Build history of the part. All positions in model axes, mm. A direction names the side the tool comes from. Round coordinates to 2 decimals unless told otherwise and drop trailing zeros. Write each loop counter-clockwise with the first axis right and the second up, starting at its lowest first coordinate (ties: lowest second). Pieces come first, ordered by that corner, then holes. Notation, with made-up numbers: (84.25, 46) -> (107.25, 46) arc R16 cw to (107.25, 70) -> close; hole circle Ø1 at (-34.75, 32). An arc over 180 degrees is marked (long way). One line per question, with ' | ' between items.
from build123d import *

# Parameters (mm, degrees)
SKETCH1_W                    = 275
SKETCH1_H                    = 33
BOSS_EXTRUDE1_DEPTH          = 12
CUT_EXTRUDE1_REACH           = 141.005
SKETCH2_R                    = 7
BOSS_EXTRUDE2_DEPTH          = 12
CUT_EXTRUDE3_REACH           = 264.774
SKETCH5_W                    = 14
SKETCH5_H                    = 6
FILLET1_R                    = 2
SKETCH17_W                   = 5
SKETCH17_H                   = 24
CUT_EXTRUDE9_DEPTH           = 6.5
CUT_EXTRUDE4_REACH           = 264.774
SKETCH6_W                    = 12
SKETCH6_H                    = 30
F_5_0_5_DIAMETER_HOLE2_D     = 5
F_5_0_5_DIAMETER_HOLE1_D     = 5
F_5_0_5_DIAMETER_HOLE1_DEPTH = 12
F_5_0_5_DIAMETER_HOLE1_TIP   = 1.502151548
FILLET2_R                    = 10
CUT_EXTRUDE5_REACH           = 264.774
CUT_EXTRUDE10_REACH          = 264.774
FILLET1_OF_MIRROR2_R         = 2


with BuildPart() as part:
    # Sketch1 → Boss-Extrude1 (new body)
    with BuildSketch(Plane.XY):
        Rectangle(SKETCH1_W, SKETCH1_H)
    extrude(amount=BOSS_EXTRUDE1_DEPTH)

    # Sketch2 → Cut-Extrude1 (cut, up to next)
    with BuildSketch(Plane.XY.offset(12), mode=Mode.PRIVATE) as cut_extrude1_sk1:
        with Locations((0, 1)):
            Circle(SKETCH2_R)
    cut_extrude1_tool1 = extrude(cut_extrude1_sk1.sketch, amount=-CUT_EXTRUDE1_REACH, mode=Mode.PRIVATE) & part.part
    add(cut_extrude1_tool1.solids().sort_by_distance((0, 1, 12))[0], mode=Mode.SUBTRACT)

    # Sketch3 → Boss-Extrude2 (add)
    with BuildSketch(Plane.XY.offset(12)):
        Polygon((-210, 16.5), (210, 16.5), (210, 157.5), (183, 157.5), (183, 46.5), (-183, 46.5), (-183, 157.5), (-210, 157.5), align=None)
    extrude(amount=-BOSS_EXTRUDE2_DEPTH)

    # Sketch5 → Cut-Extrude3 (cut, up to next)
    with BuildSketch(Plane.XY.offset(12), mode=Mode.PRIVATE) as cut_extrude3_sk1:
        with Locations((-176, 43.5)):
            Rectangle(SKETCH5_W, SKETCH5_H)
    cut_extrude3_tool1 = extrude(cut_extrude3_sk1.sketch, amount=-CUT_EXTRUDE3_REACH, mode=Mode.PRIVATE) & part.part
    # Sketch5 → Cut-Extrude3 (cut, up to next)
    with BuildSketch(Plane.XY.offset(12), mode=Mode.PRIVATE) as cut_extrude3_sk2:
        with Locations((-144, 43.5)):
            Rectangle(SKETCH5_W, SKETCH5_H)
    cut_extrude3_tool2 = extrude(cut_extrude3_sk2.sketch, amount=-CUT_EXTRUDE3_REACH, mode=Mode.PRIVATE) & part.part
    cut_extrude3_1 = cut_extrude3_tool1.solids().sort_by_distance((-176, 43.5, 12))[0]
    add(cut_extrude3_1, mode=Mode.SUBTRACT)
    cut_extrude3_2 = cut_extrude3_tool2.solids().sort_by_distance((-144, 43.5, 12))[0]
    add(cut_extrude3_2, mode=Mode.SUBTRACT)
    cut_extrude3 = cut_extrude3_1 + cut_extrude3_2  # Cut-Extrude3 as one shape, for the pattern or mirror that repeats it

    # Fillet1
    fillet1_edges = [part.edges().sort_by_distance(p)[0] for p in [
        (-169, 46.5, 6),
        (-169, 40.5, 6),
        (-183, 40.5, 6),
        (-151, 46.5, 6),
        (-137, 46.5, 6),
        (-137, 40.5, 6),
        (-151, 40.5, 6),
    ]]
    fillet(fillet1_edges, radius=FILLET1_R)

    # Sketch17 → Cut-Extrude9 (cut)
    with BuildSketch(Plane(origin=(0, 0, 0), x_dir=(-1, 0, 0), z_dir=(0, 0, -1))):
        with Locations((144, 40.5)):
            Rectangle(SKETCH17_W, SKETCH17_H)
        with Locations((176, 40.5)):
            Rectangle(SKETCH17_W, SKETCH17_H)
    cut_extrude9 = extrude(amount=-CUT_EXTRUDE9_DEPTH, mode=Mode.SUBTRACT)

    # Sketch6 → Cut-Extrude4 (cut, up to next)
    with BuildSketch(Plane.XY.offset(12), mode=Mode.PRIVATE) as cut_extrude4_sk1:
        with Locations((-194, 142.5)):
            Rectangle(SKETCH6_W, SKETCH6_H)
    cut_extrude4_tool1 = extrude(cut_extrude4_sk1.sketch, amount=-CUT_EXTRUDE4_REACH, mode=Mode.PRIVATE) & part.part
    cut_extrude4 = cut_extrude4_tool1.solids().sort_by_distance((-194, 142.5, 12))[0]
    add(cut_extrude4, mode=Mode.SUBTRACT)

    # Mirror3: Cut-Extrude4 across plane
    add(cut_extrude4.mirror(Plane(origin=(0, 0, 0), x_dir=(0, 0, 1), z_dir=(1, 0, 0))), mode=Mode.SUBTRACT)

    # Ø5.0 (5) Diameter Hole2 (through all)
    with Locations(Plane.XY.offset(12)):
        with Locations((-192, 40.5), (-192, 109.5)):
            f_5_0_5_diameter_hole2 = Hole(F_5_0_5_DIAMETER_HOLE2_D / 2)

    # Mirror4: Ø5.0 (5) Diameter Hole2 across plane
    add(f_5_0_5_diameter_hole2.mirror(Plane(origin=(0, 0, 0), x_dir=(0, 0, 1), z_dir=(1, 0, 0))), mode=Mode.SUBTRACT)

    # Ø5.0 (5) Diameter Hole1
    with Locations(Plane.XY.offset(12)):
        with Locations((-60, 24.5), (60, 24.5), (-160, 24.5), (160, 24.5)):
            Hole(F_5_0_5_DIAMETER_HOLE1_D / 2, depth=F_5_0_5_DIAMETER_HOLE1_DEPTH)
            with Locations((0, 0, -(F_5_0_5_DIAMETER_HOLE1_DEPTH + F_5_0_5_DIAMETER_HOLE1_TIP / 2))):  # 118° drill point
                Cone(0, F_5_0_5_DIAMETER_HOLE1_D / 2, F_5_0_5_DIAMETER_HOLE1_TIP, mode=Mode.SUBTRACT)

    # Fillet2
    fillet2_edges = [part.edges().sort_by_distance(p)[0] for p in [
        (210, 157.5, 6),
        (210, 16.5, 6),
        (-210, 16.5, 6),
        (-210, 157.5, 6),
    ]]
    fillet(fillet2_edges, radius=FILLET2_R - 0.0001)  # a hair under: the kernel refuses the full size

    # Sketch11 → Cut-Extrude5 (cut, up to next)
    with BuildSketch(Plane(origin=(0, 0, 0), x_dir=(-1, 0, 0), z_dir=(0, 0, -1)), mode=Mode.PRIVATE) as cut_extrude5_sk1:
        with BuildLine():
            Line((-200, 127.5), (-196, 127.5))
            ThreePointArc((-196, 127.5), (-198, 125.5), (-200, 127.5))
        make_face()
    cut_extrude5_tool1 = extrude(cut_extrude5_sk1.sketch, amount=-CUT_EXTRUDE5_REACH, mode=Mode.PRIVATE) & part.part
    # Sketch11 → Cut-Extrude5 (cut, up to next)
    with BuildSketch(Plane(origin=(0, 0, 0), x_dir=(-1, 0, 0), z_dir=(0, 0, -1)), mode=Mode.PRIVATE) as cut_extrude5_sk2:
        with BuildLine():
            Line((-192, 127.5), (-188, 127.5))
            ThreePointArc((-188, 127.5), (-190, 125.5), (-192, 127.5))
        make_face()
    cut_extrude5_tool2 = extrude(cut_extrude5_sk2.sketch, amount=-CUT_EXTRUDE5_REACH, mode=Mode.PRIVATE) & part.part
    # Sketch11 → Cut-Extrude5 (cut, up to next)
    with BuildSketch(Plane(origin=(0, 0, 0), x_dir=(-1, 0, 0), z_dir=(0, 0, -1)), mode=Mode.PRIVATE) as cut_extrude5_sk3:
        with BuildLine():
            Line((188, 127.5), (192, 127.5))
            ThreePointArc((192, 127.5), (190, 125.5), (188, 127.5))
        make_face()
    cut_extrude5_tool3 = extrude(cut_extrude5_sk3.sketch, amount=-CUT_EXTRUDE5_REACH, mode=Mode.PRIVATE) & part.part
    # Sketch11 → Cut-Extrude5 (cut, up to next)
    with BuildSketch(Plane(origin=(0, 0, 0), x_dir=(-1, 0, 0), z_dir=(0, 0, -1)), mode=Mode.PRIVATE) as cut_extrude5_sk4:
        with BuildLine():
            Line((196, 127.5), (200, 127.5))
            ThreePointArc((200, 127.5), (198, 125.5), (196, 127.5))
        make_face()
    cut_extrude5_tool4 = extrude(cut_extrude5_sk4.sketch, amount=-CUT_EXTRUDE5_REACH, mode=Mode.PRIVATE) & part.part
    add(cut_extrude5_tool1.solids().sort_by_distance((198, 126.651174, 0))[0], mode=Mode.SUBTRACT)
    add(cut_extrude5_tool2.solids().sort_by_distance((190, 126.651174, 0))[0], mode=Mode.SUBTRACT)
    add(cut_extrude5_tool3.solids().sort_by_distance((-190, 126.651174, 0))[0], mode=Mode.SUBTRACT)
    add(cut_extrude5_tool4.solids().sort_by_distance((-198, 126.651174, 0))[0], mode=Mode.SUBTRACT)

    # Sketch18 → Cut-Extrude10 (cut, up to next)
    with BuildSketch(Plane(origin=(0, 0, 0), x_dir=(-1, 0, 0), z_dir=(0, 0, -1)), mode=Mode.PRIVATE) as cut_extrude10_sk1:
        with BuildLine():
            Line((150, 16.5), (137.5, 16.5))
            Line((137.5, 16.5), (137.5, 24.5))
            ThreePointArc((137.5, 24.5), (135.5, 26.5), (137.5, 28.5))
            Line((137.5, 28.5), (150, 28.5))
            ThreePointArc((150, 28.5), (152, 26.5), (150, 24.5))
            Line((150, 24.5), (150, 16.5))
        make_face()
    cut_extrude10_tool1 = extrude(cut_extrude10_sk1.sketch, amount=-CUT_EXTRUDE10_REACH, mode=Mode.PRIVATE) & part.part
    # Sketch18 → Cut-Extrude10 (cut, up to next)
    with BuildSketch(Plane(origin=(0, 0, 0), x_dir=(-1, 0, 0), z_dir=(0, 0, -1)), mode=Mode.PRIVATE) as cut_extrude10_sk2:
        with BuildLine():
            Line((170, 16.5), (182, 16.5))
            Line((182, 16.5), (182, 24.5))
            ThreePointArc((182, 24.5), (184, 26.5), (182, 28.5))
            Line((182, 28.5), (170, 28.5))
            ThreePointArc((170, 28.5), (168, 26.5), (170, 24.5))
            Line((170, 24.5), (170, 16.5))
        make_face()
    cut_extrude10_tool2 = extrude(cut_extrude10_sk2.sketch, amount=-CUT_EXTRUDE10_REACH, mode=Mode.PRIVATE) & part.part
    cut_extrude10_1 = cut_extrude10_tool1.solids().sort_by_distance((-143.75, 22.8092, 0))[0]
    add(cut_extrude10_1, mode=Mode.SUBTRACT)
    cut_extrude10_2 = cut_extrude10_tool2.solids().sort_by_distance((-176, 22.821049, 0))[0]
    add(cut_extrude10_2, mode=Mode.SUBTRACT)
    cut_extrude10 = cut_extrude10_1 + cut_extrude10_2  # Cut-Extrude10 as one shape, for the pattern or mirror that repeats it

    # Mirror2: Cut-Extrude3, Cut-Extrude9, Cut-Extrude10 across plane
    add(cut_extrude3.mirror(Plane(origin=(0, 0, 0), x_dir=(0, 0, 1), z_dir=(1, 0, 0))), mode=Mode.SUBTRACT)
    add(cut_extrude9.mirror(Plane(origin=(0, 0, 0), x_dir=(0, 0, 1), z_dir=(1, 0, 0))), mode=Mode.SUBTRACT)
    add(cut_extrude10.mirror(Plane(origin=(0, 0, 0), x_dir=(0, 0, 1), z_dir=(1, 0, 0))), mode=Mode.SUBTRACT)

    # Fillet1 of Mirror2
    fillet1_of_mirror2_edges = [part.edges().sort_by_distance(p)[0] for p in [
        (169, 46.5, 6),
        (169, 40.5, 6),
        (183, 40.5, 6),
        (151, 46.5, 6),
        (137, 46.5, 6),
        (137, 40.5, 6),
        (151, 40.5, 6),
    ]]
    fillet(fillet1_of_mirror2_edges, radius=FILLET1_OF_MIRROR2_R)


solid = part.part
(1) Slice it at B-B (z = 2.25). State how many separate pieces and enclosed holes the cut face has, then the cut area to 3 significant figures.
Calculated:
separate pieces: 5 | enclosed holes: 9 | area: 25,300 mm2
(2) 3-axis set-ups, long thin cutter, end or side, ignore diameter. For faces 1 (the flat face through (2, 46.5, 6)), 2 (the flat face through (176, 28.5, 7)), 3 (the flat face through (-160, 16.5, 6)): which of +Z, -Z, +X, -X, +Y, -Y reach the whole face in a straight line?
Calculated:
face 1: +Z, -Z, +Y | face 2: +Z, -Z, -Y | face 3: +Z, -Z, -X, -Y
(3) Slice it at A-A (y = 1). Write the cut outline in (x, z), then the cut area to 3 significant figures.
Calculated:
outline: (-137.5, 0) -> (-7, 0) -> (-7, 12) -> (-137.5, 12) -> close; (7, 0) -> (137.5, 0) -> (137.5, 12) -> (7, 12) -> close | area: 3,130 mm2
(4) Wall check: line 1 (X direction, y = 31.5, z = 0.5); line 2 (Y direction, x = -60, z = 3.5); line 3 (Y direction, x = 0, z = 3.5). Give the ranges that are in metal, low to high. Write a range as from..to.
Calculated:
line 1: -210..-178.5, -173.5..-146.5, -141.5..141.5, 146.5..173.5, 178.5..210 | line 2: -16.5..22, 27..46.5 | line 3: -16.5..-6, 8..46.5
(5) Slice it at C-C (x = -13.5). Write the cut outline in (y, z).
Calculated:
outline: (-16.5, 0) -> (46.5, 0) -> (46.5, 12) -> (-16.5, 12) -> close
(6) Drop flat-ended pins along their axis: pin 1 (3.5 mm diameter, centred on x = 159, z = 4, fed in from +Y); pin 2 (3 mm diameter, centred on x = -194, z = 4.5, fed in from +Y); pin 3 (3 mm diameter, centred on x = 144, z = 8.5, fed in from +Y). Give the stop position or say it passes through.
Calculated:
pin 1: y = 46.5 | pin 2: y = 127.5 | pin 3: y = 40.5
(7) Mould opens along X. For faces 4 (the cylindrical face through (-207.15, 154.49, 5.92)), 5 (the flat face through (-176, 28.5, 7)), 6 (the flat face through (160, 16.5, 6)) say: pulls with the +X half, pulls with the -X half, needs draft (parallel to the pull), parting line crosses it, or undercut.
Calculated:
face 4: pulls with the -X half | face 5: undercut | face 6: needs draft
